from build123d import *

# Parameters (mm, degrees)
SKETCH1_R           = 2.075
BOSS_EXTRUDE1_DEPTH = 26.9875
SKETCH2_W           = 86.364255874
SKETCH2_H           = 34.814742066
CUT_EXTRUDE1_DEPTH  = 47.713127442


with BuildPart() as part:
    # Sketch1 → Boss-Extrude1 (new body)
    with BuildSketch(Plane.XY):
        with BuildLine():
            Line((36.087463381, 2.999957931), (36.087463381, 7.227968589))
            ThreePointArc((36.087463381, 7.227968589), (34.127671177, 11.236796761), (29.760414833, 12.152526428))
            add(Edge.make_bspline(
                [(29.760414833, 12.152526428), (20.104550549, 9.70736649), (4.160634919, 5.361227781), (-17.353300331, -1.599332571), (-25.573599276, -4.860049738), (-35.772390435, -8.549078563), (-32.029323662, -8.160268468)],
                knots=[0.330745029, 0.330745029, 0.330745029, 0.330745029, 0.630725311, 0.824213609, 0.940085477, 1, 1, 1, 1], degree=3))
            add(Edge.make_bspline(
                [(-32.029323662, -8.160268468), (-27.594277811, -7.052683566), (-20.08844374, -6.583461174), (-6.740332369, -4.760965275), (4.869732234, -4.072592428), (18.49447741, -2.742713062), (26.204740163, -2.287162162), (31.22157185, -2.075528013)],
                knots=[0, 0, 0, 0, 0.144322392, 0.237947652, 0.42712275, 0.512831912, 0.67202474, 0.67202474, 0.67202474, 0.67202474], degree=3))
            ThreePointArc((31.22157185, -2.075528013), (34.674483358, -0.515630852), (36.087463381, 2.999957931))
        make_face()
        with Locations((26.390676338, 7.079731532)):
            Circle(SKETCH1_R, mode=Mode.SUBTRACT)
    extrude(amount=BOSS_EXTRUDE1_DEPTH)

    # Sketch2 → Cut-Extrude1 (cut, through all)
    with BuildSketch(Plane.XY.offset(26.9875)):
        with Locations((-20.601451599, -3.276083686)):
            Rectangle(SKETCH2_W, SKETCH2_H)
    extrude(amount=-CUT_EXTRUDE1_DEPTH, mode=Mode.SUBTRACT)


solid = part.part
Source: CAD feature listing. Evaluate the final solid. Frame: model axes, mm. Coordinates: 2 decimals unless noted, no trailing zeros. Order: outer loops, then holes, each group sorted by start corner. A loop starts at its lowest first (then second) coordinate and runs counter-clockwise, first axis right, second up.
Item 1: Material intervals for line 1 (X direction, y = 7, z = 8.75); line 2 (Y direction, x = 26, z = 22.25); line 3 (Y direction, x = 26.75, z = 3.5), sorted ascending.
Output values:
line 1: x = 22.58 to 24.32, 28.46 to 36.09
line 2: y = -2.33 to 5.04, 9.12 to 11.19
line 3: y = -2.29 to 5.04, 9.12 to 11.38
Item 2: Cut plane A-A (y = 0). Return loops of the section in (x, z).
Output values:
outline: (22.58, 0) - (35.11, 0) - (35.11, 26.99) - (22.58, 26.99) - close
Item 3: First-contact query: P1, Ø5, axis at x = 29.5, z = 22, coming from the -Y side; P2, Ø4, axis at x = 27, z = 22.5, coming from the -Y side; P3, Ø2, axis at y = 10.5, z = 13.5, coming from the +X side. Flat tips, straight axial feed; report the tip coordinate or a pass-through.
Output values:
P1: stops at y = -2.27
P2: stops at y = -2.38
P3: stops at x = 35.55
Item 4: Pull-direction query (Y, two-part tool) for faces 1 (the face through (36.087, 5, 13)), 2 (the face through (34.178, 11.197, 13.305)), 3 (the face through (28.307, 6.285, 13.305)); classes: pulls with the +Y half, pulls with the -Y half, needs draft (parallel to the pull), parting line crosses it, or undercut.
Output values:
face 1: needs draft
face 2: pulls with the +Y half
face 3: undercut
Item 5: Cut plane B-B (x = 34.25). Return loops of the section in (y, z).
Output values:
outline: (-0.91, 0) - (11.14, 0) - (11.14, 26.99) - (-0.91, 26.99) - close
